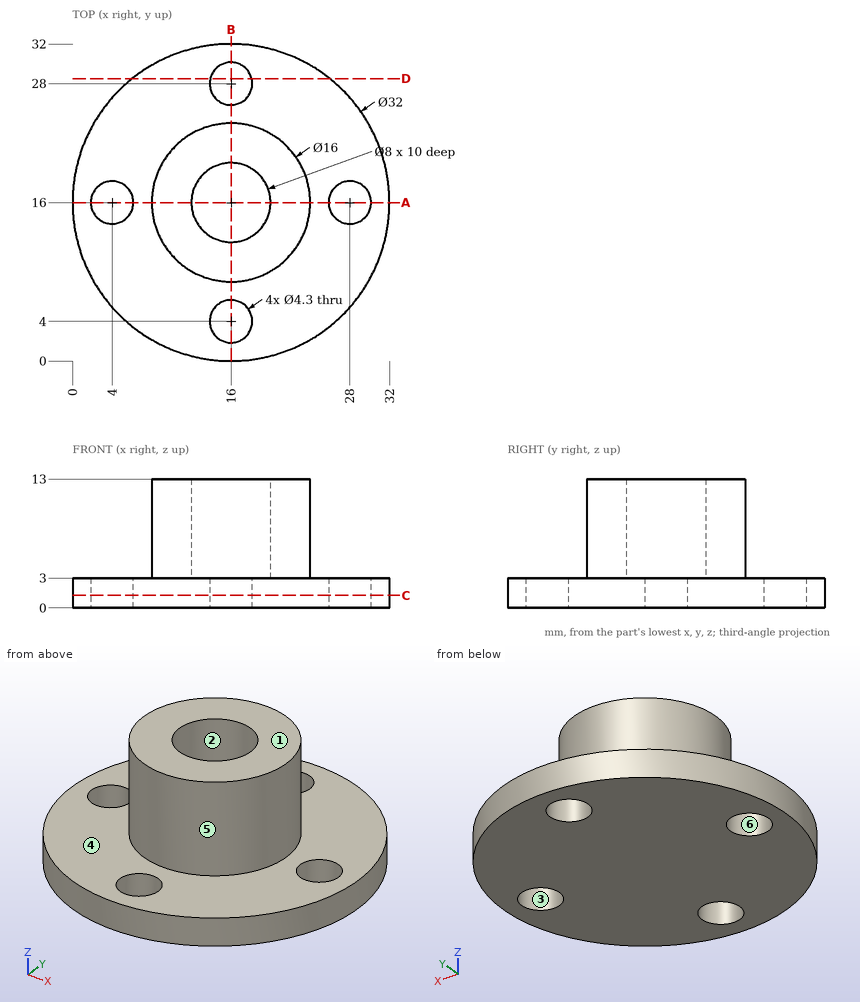
Answer from the drawing. Dimensions are ordinates in mm from the lowest x, y and z of the part. A direction names the side the tool comes from. Give positions to 0.01 mm unless a question says otherwise; leave off trailing zeros. Loops run counter-clockwise (first coordinate to the right, second up) from the corner with the lowest first, then second, coordinate; pieces in that order, holes last.
Item 1: Each of these flat-tipped pins is pushed along its axis until it touches: pin 1 Ø7 at (x, y) = (28, 16) entering from +Z; pin 2 Ø2.5 at (x, y) = (16, 4) entering from -Z. Where does it stop, or does it pass through?
Item 2: For the marked faces 1 and 2, determine the directions among +Z, -Z, +X, -X, +Y, -Y from which every point of the face is accessible in a straight line to the end or side of a thin tool.
Item 3: The mould has two halves that part along Y. Classify the marked faces 3, 4, 5 and 6: released by +Y, released by -Y, zero draft, split by the parting line, or undercut.
Item 4: Find the intervals of material crossed by line 1 along Y through (x, z) = (16, 0.85); line 2 along Y through (x, z) = (16, 8.75); line 3 along Z through (x, y) = (5, 19.5), in increasing order.
Item 5: The part is cut by section C-C (z = 1.25). Write down the section's boundary in (x, y), and give its area (3 significant figures).
Item 6: The part is cut by section D-D (y = 28.5). Write down the section's boundary in (x, z).
Item 7: The part is cut by section A-A (y = 16). Write down the section's boundary in (x, z).
Taken from the geometry:
1. pin 1: stops at z = 3
1. pin 2: passes through
2. face 1: +Z, +X, -X, +Y, -Y
2. face 2: +Z
3. face 3: undercut
3. face 4: zero draft
3. face 5: split by the parting line
3. face 6: undercut
4. line 1: y = 0 to 1.85, 6.15 to 25.85, 30.15 to 32
4. line 2: y = 8 to 12, 20 to 24
4. line 3: z = 0 to 3
5. outline: circle Ø32 at (16, 16); hole circle Ø4.3 at (4, 16); hole circle Ø4.3 at (16, 4); hole circle Ø4.3 at (16, 28); hole circle Ø4.3 at (28, 16)
5. area: 746 mm2
6. outline: (6.01, 0) - (13.91, 0) - (13.91, 3) - (6.01, 3) - close; (18.09, 0) - (25.99, 0) - (25.99, 3) - (18.09, 3) - close
7. outline: (0, 0) - (1.85, 0) - (1.85, 3) - (0, 3) - close; (6.15, 0) - (25.85, 0) - (25.85, 3) - (24, 3) - (24, 13) - (20, 13) - (20, 3) - (12, 3) - (12, 13) - (8, 13) - (8, 3) - (6.15, 3) - close; (30.15, 0) - (32, 0) - (32, 3) - (30.15, 3) - close
